Can you work these out from the drawing? Everything is in mm from the part's minimum corner. Coordinates: 2 decimals unless noted, no trailing zeros. Loops run counter-clockwise (first coordinate to the right, second up) from the corner with the lowest first, then second, coordinate; pieces in that order, holes last.
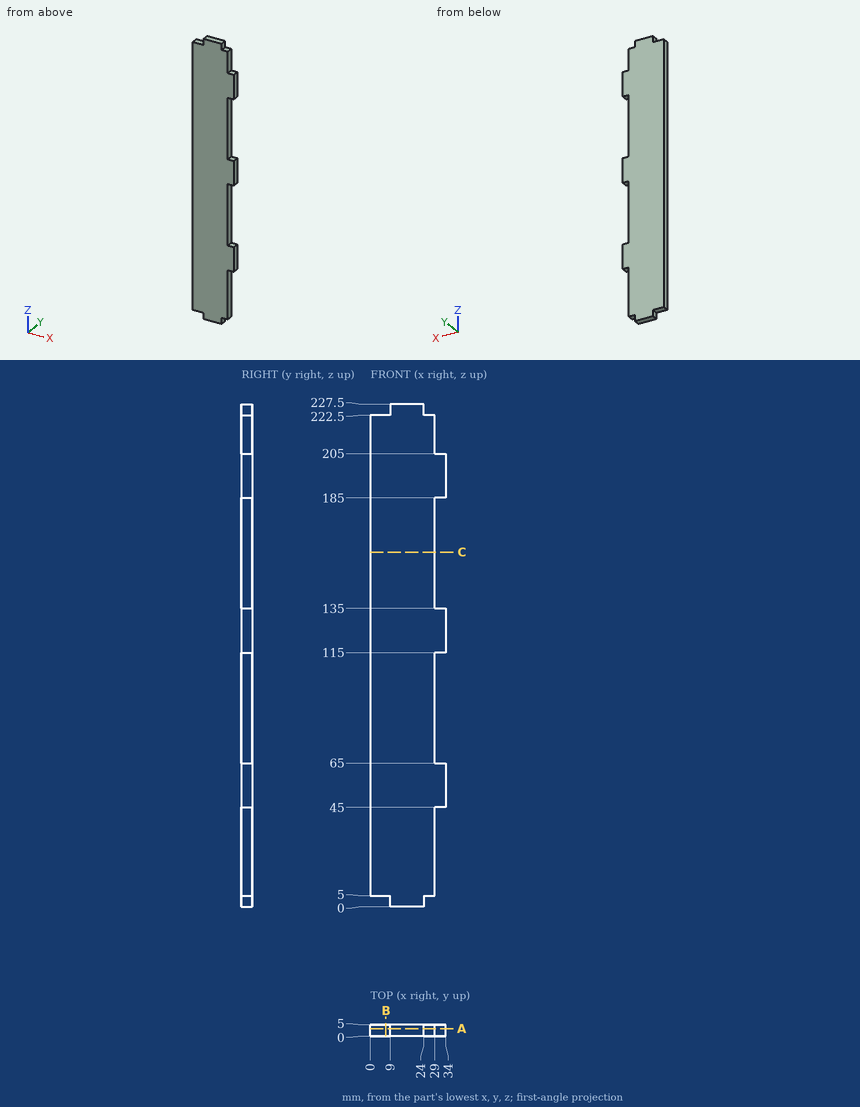
1) Imagine slicing it at A-A on y = 3.3. List the corners of the cut face in (x, z) for me, plus the area to 3 significant figures.
2) Imagine slicing it at C-C on z = 160.5. List the corners of the cut face in (x, y) for me, plus the area to 3 significant figures.
3) Imagine slicing it at B-B on x = 7. List the corners of the cut face in (y, z) for me.
4) If I drill on L1, parallel to Z at x = 31.5, y = 1.2; L2, parallel to X at y = 2.55, z = 19; L3, parallel to Z at x = 28, y = 1.05, over which ranges is the centre line in solid material (lowest first)?
5) Will these pins go through, and if not, where does the flat tip stop? pin 1 (2.5 mm diameter, centred on x = 31.5, y = 2, fed in from +Z); pin 2 (2.5 mm diameter, centred on x = 25.5, y = 3.5, fed in from -Z); pin 3 (2.5 mm diameter, centred on y = 2.5, z = 168.5, fed in from +X).
Solved:
1. outline: (0, 5) - (9, 5) - (9, 0) - (24, 0) - (24, 5) - (29, 5) - (29, 45) - (34, 45) - (34, 65) - (29, 65) - (29, 115) - (34, 115) - (34, 135) - (29, 135) - (29, 185) - (34, 185) - (34, 205) - (29, 205) - (29, 222.5) - (24, 222.5) - (24, 227.5) - (9, 227.5) - (9, 222.5) - (0, 222.5) - close
1. area: 6,760 mm2
2. outline: (0, 0) - (29, 0) - (29, 5) - (0, 5) - close
2. area: 145 mm2
3. outline: (0, 5) - (5, 5) - (5, 222.5) - (0, 222.5) - close
4. L1: z = 45 to 65, 115 to 135, 185 to 205
4. L2: x = 0 to 29
4. L3: z = 5 to 222.5
5. pin 1: stops at z = 205
5. pin 2: stops at z = 5
5. pin 3: stops at x = 29
